Part model, mm, in its own coordinate system. A direction names the side the tool comes from. Give positions to 0.01 mm unless a question says otherwise; leave off trailing zeros. Order: outer loops, then holes, each group sorted by start corner. A loop starts at its lowest first (then second) coordinate and runs counter-clockwise, first axis right, second up. Notation, with made-up numbers: M 25,12.25 L 43,12.25 A33 cw 43,43.25 Z; hole C 59.5,-17.75 d2. An arc over 180 degrees is marked long. Answer as a JSON object with one key per item and string values.
from build123d import *

# Parameters (mm, degrees)
SKETCH1_R           = 27.889608224
SKETCH1_R_2         = 3
BOSS_EXTRUDE1_DEPTH = 20
SKETCH2_R           = 26.889608224
CUT_EXTRUDE1_DEPTH  = 3
SKETCH2_5_R         = 25.031826588
SKETCH2_5_R_2       = 19.031826588
CUT_EXTRUDE2_DEPTH  = 6
FILLET1_R           = 3
SKETCH4_R           = 11.678118969
SKETCH4_R_2         = 3
BOSS_EXTRUDE2_DEPTH = 11
CHAMFER1_SIZE       = 5
SKETCH5_R           = 27.889608224
SKETCH5_R_2         = 19.009910513
CUT_EXTRUDE3_DEPTH  = 10
CHAMFER2_SIZE       = 6
CHAMFER2_SIZE2      = 4.047051101


with BuildPart() as part:
    # Sketch1 → Boss-Extrude1 (new body)
    with BuildSketch(Plane(origin=(0, 0, 0), x_dir=(1, 0, 0), z_dir=(0, 1, 0))):
        with Locations(Location((0, 0, 0), (0, 0, 270))):
            Circle(SKETCH1_R)
        with Locations(Location((0, 0, 0), (0, 0, 270))):
            Circle(SKETCH1_R_2, mode=Mode.SUBTRACT)
    extrude(amount=BOSS_EXTRUDE1_DEPTH)

    # Sketch2 → Cut-Extrude1 (cut)
    with BuildSketch(Plane(origin=(0, 20, 0), x_dir=(1, 0, 0), z_dir=(0, 1, 0))):
        with Locations(Location((0, 0, 0), (0, 0, 270))):
            Circle(SKETCH2_R)
    extrude(amount=-CUT_EXTRUDE1_DEPTH, mode=Mode.SUBTRACT)

    # Sketch2<5> → Cut-Extrude2 (cut)
    with BuildSketch(Plane(origin=(0, 20, 0), x_dir=(1, 0, 0), z_dir=(0, 1, 0))):
        with Locations(Location((0, 0, 0), (0, 0, 270))):
            Circle(SKETCH2_5_R)
        with Locations(Location((0, 0, 0), (0, 0, 270))):
            Circle(SKETCH2_5_R_2, mode=Mode.SUBTRACT)
    extrude(amount=-CUT_EXTRUDE2_DEPTH, mode=Mode.SUBTRACT)

    # Fillet1
    fillet1_edges = [part.edges().sort_by_distance(p)[0] for p in [
        (0, 14, -25.031826588),
        (0, 14, -19.031826588),
    ]]
    fillet(fillet1_edges, radius=FILLET1_R - 0.0001)  # a hair under: the kernel refuses the full size

    # Sketch4 → Boss-Extrude2 (add)
    with BuildSketch(Plane(origin=(0, 17, 0), x_dir=(1, 0, 0), z_dir=(0, 1, 0))):
        with Locations(Location((0, 0, 0), (0, 0, 270))):
            Circle(SKETCH4_R)
        with Locations(Location((0, 0, 0), (0, 0, 270))):
            Circle(SKETCH4_R_2, mode=Mode.SUBTRACT)
    extrude(amount=BOSS_EXTRUDE2_DEPTH)

    # Chamfer1
    chamfer1_edges = [part.edges().sort_by_distance(p)[0] for p in [
        (0, 28, -11.678118969),
    ]]
    chamfer(chamfer1_edges, length=CHAMFER1_SIZE)

    # Sketch5 → Cut-Extrude3 (cut)
    with BuildSketch(Plane.XZ):
        with Locations(Location((0, 0, 0), (0, 0, 270))):
            Circle(SKETCH5_R)
        with Locations(Location((0, 0, 0), (0, 0, 270))):
            Circle(SKETCH5_R_2, mode=Mode.SUBTRACT)
    extrude(amount=-CUT_EXTRUDE3_DEPTH, mode=Mode.SUBTRACT)

    # Chamfer2
    chamfer2_edges = [part.edges().sort_by_distance(p)[0] for p in [
        (0, 10, -27.889608224),
    ]]
    chamfer2_side = [part.faces().sort_by_distance(p)[0] for p in [
        (0, 10, -27.10077098),
    ]]
    chamfer(chamfer2_edges, length=CHAMFER2_SIZE, length2=CHAMFER2_SIZE2, reference=chamfer2_side[0])


solid = part.part
1. Cut at A-A on y = 7.5. Give the cut face in (x, z), plus the area to 3 significant figures.
Worked answers:
{"outline": "C 0,0 d38.02; hole C 0,0 d6", "area": "1,110 mm^2"}
2. Which spindle directions (+Z, -Z, +X, -X, +Y, -Y) get a long thin tool onto all of the face, cutting with end or side? Do faces 1 (the flat face through (-8, 17, -9)), 2 (the cylindrical face through (5.71, 4.93, -18.13)), 3 (the cylindrical face through (0.9, 13.8, 2.86)). Say none if no direction does.
Worked answers:
{"face 1": "+Y", "face 2": "-Y", "face 3": "+Y, -Y"}
3. Two-plate mould, pull along Z, no slides. Class faces 4 (the flat face through (15, 20, -23)), 5 (the flat face through (-24, 17, 8)), 6 (the conical face through (-22.075, 10.253, -2.898)): +Z half, -Z half, draft (parallel to the pull), parting line (faces both ways), or undercut.
Worked answers:
{"face 4": "draft", "face 5": "undercut", "face 6": "parting line"}
4. Pin check, flat tips, straight feed: P1, Ø8, axis at y = 10.5, z = 20.5, coming from the +X side; P2, Ø16, axis at x = -13, z = 11, coming from the +Y side; P3, Ø3, axis at x = -16, z = 10.5, coming from the +Y side. Stop position of each tip, or through.
Worked answers:
{"P1": "stops at x = 20.74", "P2": "stops at y = 25.65", "P3": "stops at y = 17"}
5. Probe line 1 along X through (y, z) = (18.05, 0); line 2 along Z through (x, y) = (-7.5, 18.25); line 3 along Y through (x, z) = (14, 11). List the from-to ranges inside material, lowest first.
Worked answers:
{"line 1": "x = -27.89 to -26.89, -11.68 to -3, 3 to 11.68, 26.89 to 27.89", "line 2": "z = -26.86 to -25.82, -8.95 to 8.95, 25.82 to 26.86", "line 3": "y = 0 to 17"}
6. Cut at B-B on y = 11.5. Give the cut face in (x, z), plus the area to 3 significant figures.
Worked answers:
{"outline": "C 0,0 d48.23; hole C 0,0 d6", "area": "1,800 mm^2"}
